Here's the drawing with two shaded views (mm, measured from the low corner). I have some questions. Give positions to 0.01 mm unless a question says otherwise; leave off trailing zeros. Write each loop counter-clockwise with the first axis right and the second up, starting at its lowest first coordinate (ties: lowest second). Pieces come first, ordered by that corner, then holes. Notation, with made-up numbers: (-25.75, -32) - (24.25, -32) arc R24 ccw to (24.25, -14) - close; hole circle Ø7 at (42, -11.5). An arc over 180 degrees is marked (long way). Write item = value, one per line.
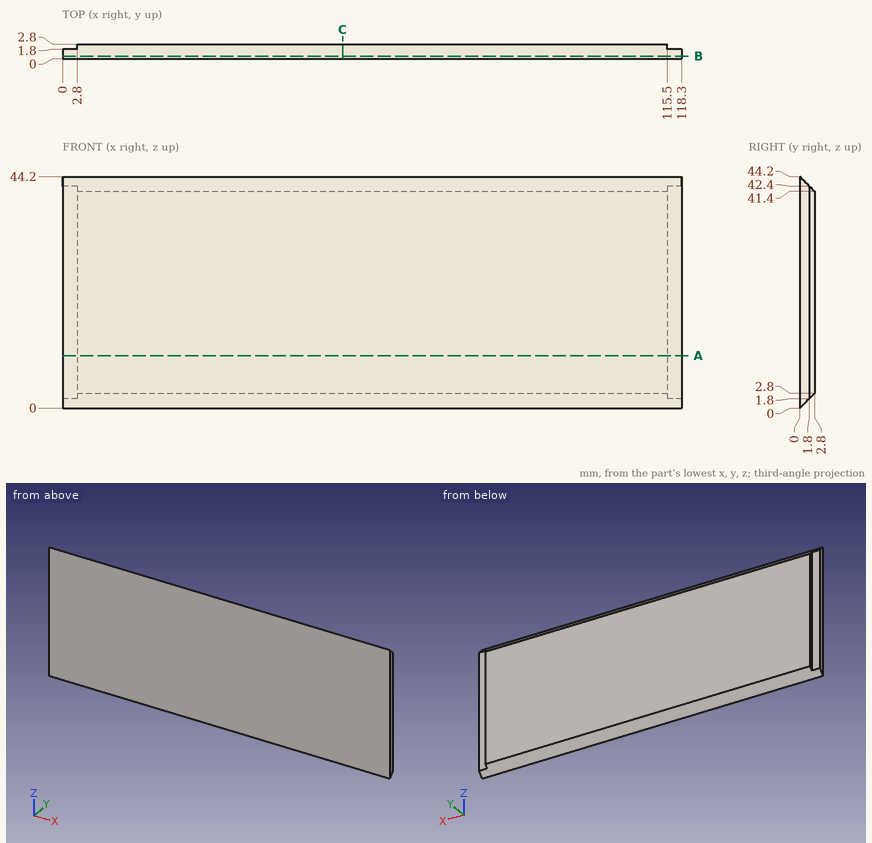
1. If we section it at C-C, the plane x = 53.5: Please give me the cut outline in (y, z).
Filled sheet:
outline = (0, 0) - (2.8, 2.8) - (2.8, 41.4) - (0, 44.2) - close
2. If we section it at B-B, the plane y = 0.5: Please give me the cut outline in (x, z).
Filled sheet:
outline = (0, 0.5) - (118.3, 0.5) - (118.3, 43.7) - (0, 43.7) - close
3. For pin 1 (1 mm diameter, centred on y = 2.5, z = 21, fed in from -X); pin 2 (1.4 mm diameter, centred on x = 117, z = 19, fed in from +Y); pin 3 (1.5 mm diameter, centred on x = 79.5, y = 0.5, fed in from +Z), each with a flat end and sliding along its axis, tell me the tip position at first contact or that it passes through.
Filled sheet:
pin_1 = 2.8
pin_2 = 1.8
pin_3 = 44.2
4. If we section it at A-A, the plane z = 10: Please give me the cut outline in (x, y).
Filled sheet:
outline = (0, 0) - (118.3, 0) - (118.3, 1.8) - (115.5, 1.8) - (115.5, 2.8) - (2.8, 2.8) - (2.8, 1.8) - (0, 1.8) - close
5. I need wall thicknesses on line 1 (X direction, y = 2.4, z = 8); line 2 (Y direction, x = 93.5, z = 41.5); line 3 (Z direction, x = 7, y = 0.5). Which ranges of each line are inside material? Lowest first, please.
Filled sheet:
line_1 = 2.8 to 115.5
line_2 = 0 to 2.7
line_3 = 0.5 to 43.7
